```python
from build123d import *

# Parameters (mm, degrees)
SKETCH1_W               = 292.1
SKETCH1_H               = 596.9
BOSS_EXTRUDE1_DEPTH     = 19.05
BOSS_EXTRUDE2_DEPTH     = 425.45
SKETCH3_W               = 25.4
SKETCH3_H               = 508
BOSS_EXTRUDE3_DEPTH     = 7.62
SKETCH4_W               = 25.4
SKETCH4_H               = 508
SKETCH4_W_2             = 15.24
SKETCH4_H_2             = 497.84
BOSS_EXTRUDE4_DEPTH     = 11.43
SKETCH5_W               = 497.84
SKETCH5_H               = 6.35
BOSS_EXTRUDE5_DEPTH     = 3.175
MIRROR2_COPY_1_SKETCH_W = 497.84
MIRROR2_COPY_1_SKETCH_H = 6.35
MIRROR2_COPY_1_DEPTH    = 3.175


with BuildPart() as part:
    # Sketch1 → Boss-Extrude1 (new body)
    with BuildSketch(Plane(origin=(0, 0, 0), x_dir=(1, 0, 0), z_dir=(0, 1, 0))):
        Rectangle(SKETCH1_W, SKETCH1_H)
    boss_extrude1 = extrude(amount=BOSS_EXTRUDE1_DEPTH)

    # Sketch2 → Boss-Extrude2 (add)
    with BuildSketch(Plane(origin=(0, 19.05, 0), x_dir=(1, 0, 0), z_dir=(0, 1, 0))):
        Polygon((-146.05, -222.25), (-146.05, 298.45), (146.05, 298.45), (146.05, -222.25), (133.35, -222.25), (133.35, 285.75), (-133.35, 285.75), (-133.35, -222.25), align=None)
    extrude(amount=BOSS_EXTRUDE2_DEPTH)

    # Sketch3 → Boss-Extrude3 (add)
    with BuildSketch(Plane(origin=(0, 19.05, 0), x_dir=(1, 0, 0), z_dir=(0, 1, 0))):
        with Locations((-82.55, -44.45)):
            Rectangle(SKETCH3_W, SKETCH3_H)
    boss_extrude3 = extrude(amount=BOSS_EXTRUDE3_DEPTH)

    # Sketch4 → Boss-Extrude4 (add)
    with BuildSketch(Plane(origin=(0, 26.67, 0), x_dir=(1, 0, 0), z_dir=(0, 1, 0))):
        with Locations((-82.55, -44.45)):
            Rectangle(SKETCH4_W, SKETCH4_H)
        with Locations((-82.55, -44.45)):
            Rectangle(SKETCH4_W_2, SKETCH4_H_2, mode=Mode.SUBTRACT)
    boss_extrude4 = extrude(amount=BOSS_EXTRUDE4_DEPTH)

    # Sketch5 → Boss-Extrude5 (add)
    with BuildSketch(Plane(origin=(-90.17, 0, 0), x_dir=(0, 0, -1), z_dir=(1, 0, 0))):
        with Locations((-44.45, 34.925)):
            Rectangle(SKETCH5_W, SKETCH5_H)
    boss_extrude5 = extrude(amount=BOSS_EXTRUDE5_DEPTH)

    # Mirror1: Boss-Extrude5 across plane
    add(boss_extrude5.mirror(Plane(origin=(-82.55, 0, 0), x_dir=(0, 0, 1), z_dir=(1, 0, 0))))

    # Mirror2: Boss-Extrude1, Boss-Extrude3, Boss-Extrude4, Boss-Extrude5 across plane
    add(boss_extrude1.mirror(Plane(origin=(0, 0, 0), x_dir=(0, 0, 1), z_dir=(1, 0, 0))))
    add(boss_extrude3.mirror(Plane(origin=(0, 0, 0), x_dir=(0, 0, 1), z_dir=(1, 0, 0))))
    add(boss_extrude4.mirror(Plane(origin=(0, 0, 0), x_dir=(0, 0, 1), z_dir=(1, 0, 0))))
    add(boss_extrude5.mirror(Plane(origin=(0, 0, 0), x_dir=(0, 0, 1), z_dir=(1, 0, 0))))

    # Mirror2 copy 1 sketch → Mirror2 copy 1 (add)
    with BuildSketch(Plane(origin=(74.93, 0, 0), x_dir=(0, 0, -1), z_dir=(1, 0, 0))):
        with Locations((-44.45, 34.925)):
            Rectangle(MIRROR2_COPY_1_SKETCH_W, MIRROR2_COPY_1_SKETCH_H)
    extrude(amount=MIRROR2_COPY_1_DEPTH)


solid = part.part
```
Part model, mm, in its own coordinate system. A direction names the side the tool comes from. Round coordinates to 2 decimals unless told otherwise and drop trailing zeros. Loops run counter-clockwise (first coordinate to the right, second up) from the corner with the lowest first, then second, coordinate; pieces in that order, holes last.
Item 1: Cut at B-B, the plane y = 82. Give the cut face in (x, z), then the cut area to 3 significant figures.
Item 2: Cut at C-C, the plane x = 40. Give the cut face in (y, z).
Item 3: Drill centre lines: line 1 (Y direction, x = 78, z = -159); line 2 (X direction, y = 367.5, z = -165); line 3 (Y direction, x = -70.5, z = -89.5). Where is each one in solid material? Low to high.
Item 4: Mould opens along X. For faces 6 (the face through (-146.05, 219, -62)), 7 (the face through (-95.25, 28, 48)), 8 (the face through (141, 444.5, -116)) say: +X half, -X half, draft (parallel to the pull), parting line (faces both ways), or undercut.
Item 5: Drop flat-ended pins along their axis: P1, Ø10, axis at x = -102.5, z = 45.5, coming from the +Y side; P2, Ø2.5, axis at x = 76.5, z = -62, coming from the -Y side; P3, Ø17, axis at x = -81.5, z = 118.5, coming from the +Y side; P4, Ø1, axis at x = -80.5, z = -186.5, coming from the +Y side. Give the stop position or say it passes through.
Item 6: 3-axis set-ups, long thin cutter, end or side, ignore diameter. For faces 1 (the face through (2, 10, 298.45)), 2 (the face through (69.85, 28, 48)), 3 (the face through (-2, 0, -4)), 4 (the face through (-83, 28, -209.55)), 5 (the face through (-83, 26.67, 41)): which of +Z, -Z, +X, -X, +Y, -Y reach the whole face in a straight line?
Item 7: Cut at A-A, the plane z = -221. Give the cut face in (x, y), then the cut area to 3 significant figures.
A:
1. outline: (-146.05, -298.45) - (146.05, -298.45) - (146.05, 222.25) - (133.35, 222.25) - (133.35, -285.75) - (-133.35, -285.75) - (-133.35, 222.25) - (-146.05, 222.25) - close
1. area: 16,600 mm2
2. outline: (0, -298.45) - (444.5, -298.45) - (444.5, -285.75) - (19.05, -285.75) - (19.05, 298.45) - (0, 298.45) - close
3. line 1: y = 0 to 26.67, 31.75 to 38.1
3. line 2: x = -146.05 to -133.35, 133.35 to 146.05
3. line 3: y = 0 to 38.1
4. face 6: -X half
4. face 7: undercut
4. face 8: draft
5. P1: stops at y = 19.05
5. P2: stops at y = 0
5. P3: stops at y = 38.1
5. P4: stops at y = 26.67
6. face 1: +Z, +X, -X, +Y, -Y
6. face 2: +Z, +Y
6. face 3: +Z, -Z, +X, -X, -Y
6. face 4: +Y
6. face 5: none
7. outline: (-146.05, 0) - (146.05, 0) - (146.05, 444.5) - (133.35, 444.5) - (133.35, 19.05) - (-133.35, 19.05) - (-133.35, 444.5) - (-146.05, 444.5) - close
7. area: 16,400 mm2
